Read the model definition and answer for the solid it produces. Units are mm, in the model's axes. A direction names the side the tool comes from. Coordinates: 2 decimals unless noted, no trailing zeros. Write each loop counter-clockwise with the first axis right and the second up, starting at its lowest first coordinate (ties: lowest second). Pieces come first, ordered by that corner, then holes.
1) The part is cut by section D-D (y = -41). Determine the outline of the cut face in (x, z), then the cut area to 4 significant figures.
2) The part is cut by section A-A (x = -6). Determine the outline of the cut face in (y, z).
3) Which of the six approach directions +Z, -Z, +X, -X, +Y, -Y give full straight-line access (tool end or side, diameter ignored) to faces 4 (the face through (-2, 41, 51)), 5 (the face through (2, -41, 51)), 6 (the face through (149.3, -32.5, 25.9)), 7 (the face through (-2, -32, 25))?
4) Each of these flat-tipped pins is pushed along its axis until it touches: pin 1 Ø1 at (x, z) = (-110.5, 42) entering from +Y; pin 2 Ø1.6 at (y, z) = (37.5, 50.5) entering from +X; pin 3 Ø2 at (x, z) = (-72.5, 10) entering from -Y. Where does it stop, or does it pass through?
5) The part is cut by section B-B (y = -18.5). Determine the outline of the cut face in (x, z), then the cut area to 3 significant figures.
6) Determine the mould class of faces 1 (the face through (-158, 0, 52)), 2 (the face through (148.5, -32.3, 25.9)), 3 (the face through (150, -1, 25)) for opening direction X: +X half, -X half, draft (parallel to the pull), parting line (faces both ways), or undercut.
7) The part is cut by section C-C (z = 27.5). Determine the outline of the cut face in (x, y), then the cut area to 3 significant figures.
8) Find the intervals of material crossed by line 1 (Y direction, x = -5, z = 8); line 2 (X direction, y = -14.5, z = 18); line 3 (Z direction, x = 27.5, y = -34.5), in increasing order.
from build123d import *

# Parameters (mm, degrees)
SKETCH1_W                 = 300
SKETCH1_H                 = 66
SKETCH1_W_2               = 298
SKETCH1_H_2               = 64
BOSS_EXTRUDE1_DEPTH       = 50
CONVERT_SOLID1_DEPTH      = 50
CONVERT_SOLID1_2_DEPTH    = 50
EDGE_FLANGE1_DEPTH        = 296
EDGE_FLANGE1_BEND_DEPTH   = 63.5
EDGE_FLANGE1_BEND_2_DEPTH = 296.5
EDGE_FLANGE1_BEND_3_DEPTH = 62


# Read off the part's stored shape, not the designer's step: Convert-Solid1
# Sheet-metal steps are written as plain solids
with BuildPart() as part:
    # Sketch1 → Boss-Extrude1 (new body)
    with BuildSketch(Plane.XY):
        Rectangle(SKETCH1_W, SKETCH1_H)
        Rectangle(SKETCH1_W_2, SKETCH1_H_2, mode=Mode.SUBTRACT)
    extrude(amount=BOSS_EXTRUDE1_DEPTH)

    # Convert-Solid1 outline → Convert-Solid1 (cut)
    with BuildSketch(Plane.XY):
        Polygon((149, -32.5), (149, -32), (148.5, -32), (148.5, -33), (150, -33), (150, -32.5), align=None)
        with BuildLine():
            ThreePointArc((148, 33), (149.414213562, 32.414213562), (150, 31))
            Line((150, 31), (150, 33))
            Line((150, 33), (148, 33))
        make_face()
        with BuildLine():
            Line((-150, -33), (-148, -33))
            ThreePointArc((-148, -33), (-149.414213562, -32.414213562), (-150, -31))
            Line((-150, -31), (-150, -33))
        make_face()
        with BuildLine():
            ThreePointArc((-150, 31), (-149.414213562, 32.414213562), (-148, 33))
            Line((-148, 33), (-150, 33))
            Line((-150, 33), (-150, 31))
        make_face()
    extrude(amount=CONVERT_SOLID1_DEPTH, mode=Mode.SUBTRACT)

    # Convert-Solid1 2 outline → Convert-Solid1 2 (add)
    with BuildSketch(Plane.XY):
        with BuildLine():
            ThreePointArc((148, 32), (148.707106781, 31.707106781), (149, 31))
            Line((149, 31), (149, 32))
            Line((149, 32), (148, 32))
        make_face()
        with BuildLine():
            ThreePointArc((-149, 31), (-148.707106781, 31.707106781), (-148, 32))
            Line((-148, 32), (-149, 32))
            Line((-149, 32), (-149, 31))
        make_face()
        with BuildLine():
            Line((-149, -32), (-148, -32))
            ThreePointArc((-148, -32), (-148.707106781, -31.707106781), (-149, -31))
            Line((-149, -31), (-149, -32))
        make_face()
    extrude(amount=CONVERT_SOLID1_2_DEPTH)

    # Edge-Flange1 section (across the edge) → Edge-Flange1 (add)
    with BuildSketch(Plane(origin=(-148, 33, 51), x_dir=(0, 0, -1), z_dir=(1, 0, 0))):
        with BuildLine():
            Line((-1, 1), (-1, 15))
            Line((-1, 15), (0, 15))
            Line((0, 15), (0, 1))
            ThreePointArc((0, 1), (0.292893219, 0.292893219), (1, 0))
            Line((1, 0), (1, -1))
            ThreePointArc((1, -1), (-0.414213562, -0.414213562), (-1, 1))
        make_face()
    extrude(amount=EDGE_FLANGE1_DEPTH)

    # Edge-Flange1 section 2 (across the edge) → Edge-Flange1 bend (add)
    with BuildSketch(Plane(origin=(150, 31, 51), x_dir=(0, 0, -1), z_dir=(0, -1, 0))):
        with BuildLine():
            Line((-1, 1), (-1, 15))
            Line((-1, 15), (0, 15))
            Line((0, 15), (0, 1))
            ThreePointArc((0, 1), (0.292893219, 0.292893219), (1, 0))
            Line((1, 0), (1, -1))
            ThreePointArc((1, -1), (-0.414213562, -0.414213562), (-1, 1))
        make_face()
    extrude(amount=EDGE_FLANGE1_BEND_DEPTH)

    # Edge-Flange1 section 3 (across the edge) → Edge-Flange1 bend 2 (add)
    with BuildSketch(Plane(origin=(148.5, -33, 51), x_dir=(0, 0, -1), z_dir=(-1, 0, 0))):
        with BuildLine():
            Line((-1, 1), (-1, 15))
            Line((-1, 15), (0, 15))
            Line((0, 15), (0, 1))
            ThreePointArc((0, 1), (0.292893219, 0.292893219), (1, 0))
            Line((1, 0), (1, -1))
            ThreePointArc((1, -1), (-0.414213562, -0.414213562), (-1, 1))
        make_face()
    extrude(amount=EDGE_FLANGE1_BEND_2_DEPTH)

    # Edge-Flange1 section 4 (across the edge) → Edge-Flange1 bend 3 (add)
    with BuildSketch(Plane(origin=(-150, -31, 51), x_dir=(0, 0, -1), z_dir=(0, 1, 0))):
        with BuildLine():
            Line((-1, 1), (-1, 15))
            Line((-1, 15), (0, 15))
            Line((0, 15), (0, 1))
            ThreePointArc((0, 1), (0.292893219, 0.292893219), (1, 0))
            Line((1, 0), (1, -1))
            ThreePointArc((1, -1), (-0.414213562, -0.414213562), (-1, 1))
        make_face()
    extrude(amount=EDGE_FLANGE1_BEND_3_DEPTH)


solid = part.part
Reported:
1. outline: (-148, 51) - (148.5, 51) - (148.5, 52) - (-148, 52) - close
1. area: 296.5 mm2
2. outline: (-48, 51) - (-34, 51) arc R1 cw to (-33, 50) - (-33, 0) - (-32, 0) - (-32, 50) arc R2 ccw to (-34, 52) - (-48, 52) - close; (32, 0) - (33, 0) - (33, 50) arc R1 cw to (34, 51) - (48, 51) - (48, 52) - (34, 52) arc R2 ccw to (32, 50) - close
3. face 4: -Z, +X, -X, +Y
3. face 5: -Z, +X, -X, -Y
3. face 6: +Z, -Z, +X, -Y
3. face 7: +Z, -Z
4. pin 1: stops at y = 33
4. pin 2: stops at x = 148
4. pin 3: stops at y = -33
5. outline: (-165, 51) - (-151, 51) arc R1 cw to (-150, 50) - (-150, 0) - (-149, 0) - (-149, 50) arc R2 ccw to (-151, 52) - (-165, 52) - close; (149, 0) - (150, 0) - (150, 50) arc R1 cw to (151, 51) - (165, 51) - (165, 52) - (151, 52) arc R2 ccw to (149, 50) - close
5. area: 133 mm2
6. face 1: draft
6. face 2: undercut
6. face 3: +X half
7. outline: (-150, -31) arc R2 ccw to (-148, -33) - (148.5, -33) - (148.5, -32) - (-148, -32) arc R1 cw to (-149, -31) - (-149, 31) arc R1 cw to (-148, 32) - (148, 32) arc R1 cw to (149, 31) - (149, -32.5) - (150, -32.5) - (150, 31) arc R2 ccw to (148, 33) - (-148, 33) arc R2 ccw to (-150, 31) - close
7. area: 725 mm2
8. line 1: y = -33 to -32, 32 to 33
8. line 2: x = -150 to -149, 149 to 150
8. line 3: z = 51 to 52
